from build123d import *

# Parameters (mm, degrees)
SKETCH1_W           = 152.4
SKETCH1_H           = 12.7
BOSS_EXTRUDE1_DEPTH = 6.35
SKETCH2_R           = 1.27
CUT_EXTRUDE1_DEPTH  = 7.35
LPATTERN1_COUNT     = 12
LPATTERN1_PITCH     = 6.35
LPATTERN1_COL_COUNT = 12
LPATTERN1_COL_PITCH = 6.35
CHAMFER1_SIZE       = 6.35
FILLET1_R           = 5.08


with BuildPart() as part:
    # Sketch1 → Boss-Extrude1 (new body)
    with BuildSketch(Plane.XY):
        Rectangle(SKETCH1_W, SKETCH1_H)
    extrude(amount=BOSS_EXTRUDE1_DEPTH)

    # Sketch2 → Cut-Extrude1 (cut, through all)
    with BuildSketch(Plane.XY.offset(6.35)):
        Circle(SKETCH2_R)
    cut_extrude1 = extrude(amount=-CUT_EXTRUDE1_DEPTH, mode=Mode.SUBTRACT)

    # LPattern1: Cut-Extrude1 ×12
    with Locations(*[(i * LPATTERN1_PITCH, 0, 0) for i in range(1, LPATTERN1_COUNT)]):
        add(cut_extrude1, mode=Mode.SUBTRACT)

    # LPattern1 col: Cut-Extrude1 ×12
    with Locations(*[(-i * LPATTERN1_COL_PITCH, 0, 0) for i in range(1, LPATTERN1_COL_COUNT)]):
        add(cut_extrude1, mode=Mode.SUBTRACT)

    # Chamfer1
    chamfer1_edges = [part.edges().sort_by_distance(p)[0] for p in [
        (-76.2, 6.35, 3.175),
        (76.2, 6.35, 3.175),
    ]]
    chamfer(chamfer1_edges, length=CHAMFER1_SIZE)

    # Fillet1
    fillet1_edges = [part.edges().sort_by_distance(p)[0] for p in [
        (-69.85, 6.35, 3.175),
        (69.85, 6.35, 3.175),
        (76.2, 0, 3.175),
        (-76.2, 0, 3.175),
    ]]
    fillet(fillet1_edges, radius=FILLET1_R)


solid = part.part
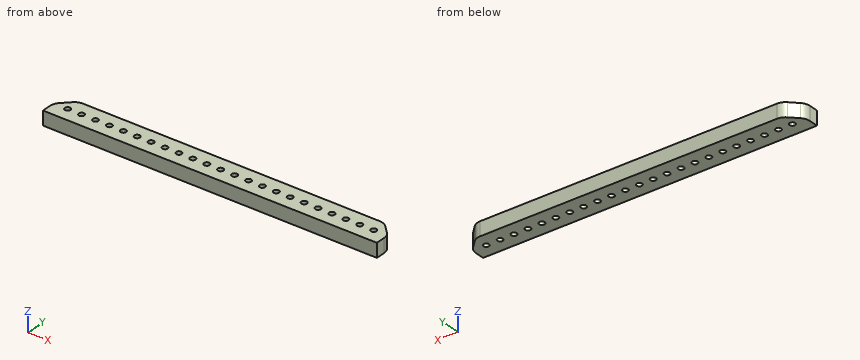
Work out the finished part from the listing and answer in its coordinate system (mm). Coordinates: 2 decimals unless noted, no trailing zeros. Write each loop counter-clockwise with the first axis right and the second up, starting at its lowest first coordinate (ties: lowest second). Pieces come first, ordered by that corner, then holes. Notation, with made-up numbers: (33, -9) - (58, -9) arc R19 cw to (58, 10) - close; hole circle Ø8 at (23, -5). An arc over 180 degrees is marked (long way). One line per question, with ' | ' between items.
1) Consider probe 1 along Y at (x, z) = (-50.8, 4); probe 2 along X at (y, z) = (-1.75, 1); probe 3 along X at (y, z) = (3.25, 5.5). Determine where each line is inside the solid, lowest interval first. Write a range as [from, to].
Checks:
probe 1: [-6.35, -1.27], [1.27, 6.35] | probe 2: [-76.19, 76.19] | probe 3: [-72.95, 72.95]
2) Find section B-B, the plane z = 5.25. Give the number of separate pieces and of enclosed holes in the cut face, and give its area (3 significant figures).
Checks:
separate pieces: 1 | enclosed holes: 23 | area: 1,780 mm2
3) Find section C-C, the plane y = 3. Determine the outline of the cut face in (x, z), and give its area (3 significant figures).
Checks:
outline: (-73.2, 0) - (73.2, 0) - (73.2, 6.35) - (-73.2, 6.35) - close | area: 930 mm2
4) Flat-ended cylindrical pins translate along their axes: P1, Ø1.5, axis at x = -57.15, y = 0, coming from the -Z side; P2, Ø3, axis at y = 3.5, z = 2, coming from the -X side. Find the tip coordinate at first contact, or state that the pin passes through.
Checks:
P1: through | P2: x = -74.2
5) Find section A-A, the plane x = 6.35. Determine the outline of the cut face in (y, z).
Checks:
outline: (-6.35, 0) - (-1.27, 0) - (-1.27, 6.35) - (-6.35, 6.35) - close; (1.27, 0) - (6.35, 0) - (6.35, 6.35) - (1.27, 6.35) - close
